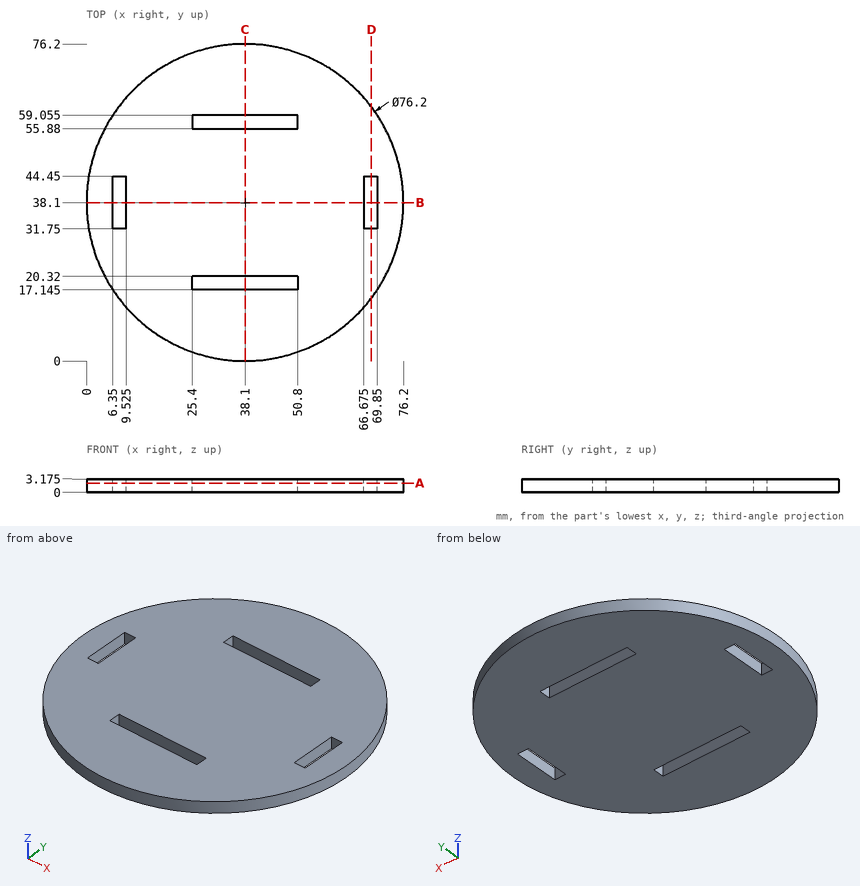
The drawing under review shows one solid part. Ordinate dimensions are in mm from its lowest x, y, z. Give positions to 0.01 mm unless a question says otherwise; leave off trailing zeros. Write each loop counter-clockwise with the first axis right and the second up, starting at its lowest first coordinate (ties: lowest second). Pieces come first, ordered by that corner, then holes. Notation, with made-up numbers: (86, 11.25) - (108, 11.25) arc R23 ccw to (108, 30.25) - close; hole circle Ø10 at (3.5, -21.5). An arc over 180 degrees is marked (long way). Answer in a Markdown table with one row per item. Add a question column.
1. Insertion check: P1, Ø1, axis at y = 58, z = 1, coming from the -X side; P2, Ø1, axis at x = 41, z = 2, coming from the -Y side; P3, Ø1, axis at y = 45, z = 1.5, coming from the -X side; P4, Ø2, axis at x = 57.5, y = 62, coming from the -Z side. Each pin has a flat end and moves straight along its axis. Give the tip position at first contact, or say it passes through.
2. We need section C-C on x = 38.1. Write out the cut boundary in (y, z) (3 decimals).
3. We need section A-A on z = 2.2. Write out the cut boundary in (x, y) (3 decimals), then the cut area to 3 significant figures.
4. We need section B-B on y = 38.1. Write out the cut boundary in (x, z) (3 decimals).
5. We need section D-D on x = 68.5. Write out the cut boundary in (y, z) (3 decimals), then the cut area to 3 significant figures.
6. Wall thickness on line 1 along X through (y, z) = (37.5, 0.85) (3 decimals); line 2 along Y through (x, z) = (46.5, 1.2) (3 decimals); line 3 along Y through (x, z) = (49, 0.9) (3 decimals): over which ranges is each line inside the solid? List them lowest first. Write a range as [from, to].
Ans:
| question | item | result |
|---|---|---|
| 1 | P1 | stops at x = 5.31 |
| 1 | P2 | stops at y = 0.08 |
| 1 | P3 | stops at x = 0.54 |
| 1 | P4 | stops at z = 0 |
| 2 | outline | (0, 0) - (17.145, 0) - (17.145, 3.175) - (0, 3.175) - close; (20.32, 0) - (55.88, 0) - (55.88, 3.175) - (20.32, 3.175) - close; (59.055, 0) - (76.2, 0) - (76.2, 3.175) - (59.055, 3.175) - close |
| 3 | outline | circle Ø76.2 at (38.1, 38.1); hole (6.35, 31.75) - (9.525, 31.75) - (9.525, 44.45) - (6.35, 44.45) - close; hole (25.4, 17.145) - (50.8, 17.145) - (50.8, 20.32) - (25.4, 20.32) - close; hole (25.4, 55.88) - (50.8, 55.88) - (50.8, 59.055) - (25.4, 59.055) - close; hole (66.675, 31.75) - (69.85, 31.75) - (69.85, 44.45) - (66.675, 44.45) - close |
| 3 | area | 4,320 mm^2 |
| 4 | outline | (0, 0) - (6.35, 0) - (6.35, 3.175) - (0, 3.175) - close; (9.525, 0) - (66.675, 0) - (66.675, 3.175) - (9.525, 3.175) - close; (69.85, 0) - (76.2, 0) - (76.2, 3.175) - (69.85, 3.175) - close |
| 5 | outline | (15.134, 0) - (31.75, 0) - (31.75, 3.175) - (15.134, 3.175) - close; (44.45, 0) - (61.066, 0) - (61.066, 3.175) - (44.45, 3.175) - close |
| 5 | area | 106 mm^2 |
| 6 | line 1 | x = [0.005, 6.35], [9.525, 66.675], [69.85, 76.195] |
| 6 | line 2 | y = [0.938, 17.145], [20.32, 55.88], [59.055, 75.262] |
| 6 | line 3 | y = [1.592, 17.145], [20.32, 55.88], [59.055, 74.608] |
